Geometry: final body of the model. Coordinates: model frame, mm. Face numbers are marked on the shaded views. A direction names the side the tool comes from. Give positions to 0.01 mm unless a question says otherwise; leave off trailing zeros. Loops run counter-clockwise (first coordinate to the right, second up) from the corner with the lowest first, then second, coordinate; pieces in that order, holes last.
1. First-contact query: P1, Ø6, axis at x = -6, y = 8, coming from the -Z side; P2, Ø8, axis at x = 69.5, z = -4, coming from the -Y side; P3, Ø7.5, axis at x = -27, z = -1.5, coming from the +Y side; P4, Ø8, axis at x = -10, y = -23.5, coming from the -Z side. Flat tips, straight axial feed; report the tip coordinate or a pass-through.
2. Section D-D, the plane y = -26. Output: boundary loops of the cut face in (x, z).
3. Section A-A, the plane z = -9. Output: boundary loops of the cut face in (x, y).
4. Section B-B, the plane y = -12. Output: boundary loops of the cut face in (x, z).
5. Material intervals for line 1 along Y through (x, z) = (-27, -3.5); line 2 along Z through (x, y) = (30, 6); line 3 along X through (y, z) = (-6, 5.75), sorted ascending.
6. Access query for the marked faces 1, 2 and 3. Directions: +Z, -Z, +X, -X, +Y, -Y. A direction counts if a zero-diameter tool reaches every point of the face in a straight line with its end or side. Return the directions, or none.
7. Section C-C, the plane x = 64. Output: boundary loops of the cut face in (y, z).
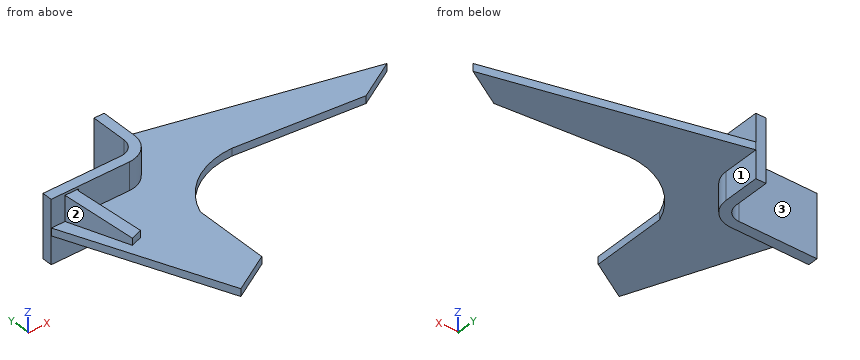
from build123d import *

# Parameters (mm, degrees)
F1_DEPTH = 1.5
F3_DEPTH = 1.5
F5_DEPTH = 12.5
F7_DEPTH = 10
F9_DEPTH = 5


with BuildPart() as f1:
    # F0 (on Top) → F1 (new body, symmetric)
    with BuildSketch(Plane.XY):
        with BuildLine():
            Line((93.483799182, 1.5717417002), (0, 24.639101699))
            Line((0, 24.639101699), (0, 10))
            ThreePointArc((0, 10), (-2.9289321881, 2.9289321881), (-10, 0))
            Line((-10, 0), (-25.5, 0))
            Line((-25.5, 0), (-41, 0))
            Line((-41, 0), (-15.5884572681, -61.4011549224))
            Line((-15.5884572681, -61.4011549224), (0, -52.4011549224))
            Line((0, -52.4011549224), (0, -22.3483927548))
            ThreePointArc((0, -22.3483927548), (11.1050484965, -8.0156356733), (28.4436228876, -2.7124417533))
            Line((28.4436228876, -2.7124417533), (77.8953419139, -7.4282582998))
            Line((77.8953419139, -7.4282582998), (93.483799182, 1.5717417002))
        make_face()
        with BuildLine():
            Line((0, 10), (0, 24.639101699))
            Line((0, 24.639101699), (-4, 24.639101699))
            Line((-4, 24.639101699), (-4, 10))
            ThreePointArc((-4, 10), (-5.7573593129, 5.7573593129), (-10, 4))
            Line((-10, 4), (-41, 4))
            Line((-41, 4), (-41, 0))
            Line((-41, 0), (-25.5, 0))
            Line((-25.5, 0), (-10, 0))
            ThreePointArc((-10, 0), (-2.9289321881, 2.9289321881), (0, 10))
        make_face()
    extrude(amount=F1_DEPTH, both=True)

    # F2 (on Top) → F3 (join, symmetric)
    with BuildSketch(Plane.XY):
        Polygon((-0.4887568886, 8.2661984248), (-11.5621451159, 1.5826697675), (-0.9085235181, -15.3436513582), (9.5235692223, -9.0471873172), align=None)
    extrude(amount=F3_DEPTH, both=True)

    # F4 (on Top) → F5 (join, symmetric)
    with BuildSketch(Plane.XY):
        with BuildLine():
            Line((-0.0799827916, 10.0108882828), (-0.0799827916, 24.6499899817))
            Line((-0.0799827916, 24.6499899817), (-4.0799827916, 24.6499899817))
            Line((-4.0799827916, 24.6499899817), (-4.0799827916, 10.0108882828))
            ThreePointArc((-4.0799827916, 10.0108882828), (-5.8373421045, 5.7682475956), (-10.0799827916, 4.0108882828))
            Line((-10.0799827916, 4.0108882828), (-41.0799827916, 4.0108882828))
            Line((-41.0799827916, 4.0108882828), (-41.0799827916, 0.0108882828))
            Line((-41.0799827916, 0.0108882828), (-10.0799827916, 0.0108882828))
            ThreePointArc((-10.0799827916, 0.0108882828), (-3.0089149798, 2.9398204709), (-0.0799827916, 10.0108882828))
        make_face()
    extrude(amount=F5_DEPTH, both=True)

    # F6 (on face) → F7 (join)
    with BuildSketch(Plane.XY.offset(1.5)):
        Polygon((-35.8013698642, 0.5949702468), (-27.2878240943, -22.7958045155), (-22.773043412, -21.1525587329), (-31.2865891819, 2.2382160294), align=None)
    extrude(amount=F7_DEPTH)

    # F8 (on face) → F9 (cut)
    with BuildSketch(Plane(origin=(-31.422185401, -11.4367401815, 0), x_dir=(0.3420201433, -0.9396926208, 0), z_dir=(-0.9396926208, -0.3420201433, 0))):
        Polygon((-12.1823117593, 11.5), (12.0880637803, 4.2156488635), (12.0880637803, 11.5), align=None)
    extrude(amount=-F9_DEPTH, mode=Mode.SUBTRACT)


solid = f1.part
Answers below:
1. P1: stops at z = -12.5
1. P2: stops at y = -6.93
1. P3: stops at y = 4.01
1. P4: stops at z = -1.5
2. outline: (-30.24, -1.5) - (0, -1.5) - (0, 1.5) - (-30.24, 1.5) - close
3. outline: (-41.08, 0.01) - (-10.08, 0.01) arc R10 ccw to (-0.08, 10.01) - (-0.08, 24.65) - (-4.08, 24.65) - (-4.08, 10.01) arc R6 cw to (-10.08, 4.01) - (-41.08, 4.01) - close
4. outline: (-36.03, -1.5) - (6.44, -1.5) - (6.44, 1.5) - (-26.1, 1.5) - (-26.1, 7.14) - (-31.22, 7.66) - (-31.22, 1.5) - (-36.03, 1.5) - close
5. line 1: y = 0.01 to 4.01
5. line 2: z = -1.5 to 1.5
5. line 3: x = -33.4 to -28.29
6. face 1: +X, +Y, -Y
6. face 2: +Z, -X, -Y
6. face 3: +Z, -Z, -X, +Y
7. outline: (-6.1, -1.5) - (8.85, -1.5) - (8.85, 1.5) - (-6.1, 1.5) - close
